The listing builds one solid part. Answer for the finished solid, in the listing's coordinates (mm). Coordinates: 2 decimals unless noted, no trailing zeros. Order: outer loops, then holes, each group sorted by start corner. A loop starts at its lowest first (then second) coordinate and runs counter-clockwise, first axis right, second up.
Autodesk Inventor part; units mm, degrees
ref_plane "YZ Plane" through (0, 0, 0) normal (1, 0, 0) x (0, 1, 0)
ref_plane "XZ Plane" through (0, 0, 0) normal (0, 1, 0) x (-1, 0, 0)
ref_plane "XY Plane" through (0, 0, 0) normal (0, 0, 1) x (1, 0, 0)
sketch "Sketch1" plane through (0, 0, 0) normal (0, 1, 0) x (-1, 0, 0)
  line L0 (0, 0) -> (-140, 0)
  line L1 (-140, 0) -> (-140, -120)
  line L2 (-140, -120) -> (0, -120)
  line L3 (0, -120) -> (0, 0)
  line L4 (-25, 0) -> (-75, 0)
  line L5 (-75, 0) -> (-75, -20)
  line L6 (-75, -20) -> (-25, -20)
  line L7 (-25, -20) -> (-25, 0)
  circle A0 centre (-5, -5) radius 1.6
  circle A1 centre (-10, -5) radius 1.6
  circle A2 centre (-15, -5) radius 1.6
  circle A3 centre (-20, -5) radius 1.6
  circle A4 centre (-130, -30) radius 1.6
  line L8 (0, -60) -> (-140, -60) construction
  line L9 (-70, -120) -> (-70, 0) construction
  circle A5 centre (-135, -5) radius 1.6
  circle A6 centre (-130, -5) radius 1.6
  circle A7 centre (-125, -5) radius 1.6
  circle A8 centre (-120, -5) radius 1.6
  circle A9 centre (-130, -60) radius 1.6
  circle A10 centre (-130, -30) radius 2.75
  circle A11 centre (-130, -60) radius 2.75
  circle A12 centre (-5, -115) radius 1.6
  circle A13 centre (-10, -115) radius 1.6
  circle A14 centre (-30, -110) radius 1.6
  circle A15 centre (-30, -110) radius 2.75
  circle A16 centre (-110, -110) radius 1.6
  circle A17 centre (-110, -110) radius 2.75
  circle A18 centre (-70, -110) radius 1.6
  circle A19 centre (-70, -110) radius 2.75
  circle A20 centre (-44, -38) radius 1.6
  circle A21 centre (-44, -38) radius 2.75
  circle A22 centre (-56, -38) radius 1.6
  circle A23 centre (-56, -38) radius 2.75
  circle A24 centre (-57.5, -60) radius 1.6
  circle A25 centre (-57.5, -60) radius 2.75
  circle A26 centre (-57.5, -72) radius 1.6
  circle A27 centre (-57.5, -72) radius 2.75
  circle A28 centre (-42.5, -60) radius 1.6
  circle A29 centre (-42.5, -60) radius 2.75
  circle A30 centre (-42.5, -72) radius 1.6
  circle A31 centre (-42.5, -72) radius 2.75
  circle A32 centre (-10, -30) radius 1.6
  circle A33 centre (-10, -60) radius 1.6
  circle A34 centre (-10, -30) radius 2.75
  circle A35 centre (-10, -60) radius 2.75
  circle A36 centre (-10, -90) radius 1.6
  circle A37 centre (-10, -90) radius 2.75
  circle A38 centre (-80, -2.5) radius 1.6
  circle A39 centre (-80, -17.5) radius 1.6
  circle A40 centre (-105, -10) radius 1.6
  circle A41 centre (-105, -20) radius 1.6
  circle A42 centre (-95, -20) radius 1.6
  circle A43 centre (-95, -10) radius 1.6
  circle A44 centre (-95, -30) radius 1.6
  circle A45 centre (-95, -40) radius 1.6
  circle A46 centre (-105, -30) radius 1.6
  circle A47 centre (-105, -40) radius 1.6
  circle A48 centre (-95, -50) radius 1.6
  circle A49 centre (-95, -60) radius 1.6
  circle A50 centre (-105, -50) radius 1.6
  circle A51 centre (-105, -60) radius 1.6
  circle A52 centre (-110, -80) radius 1.65
  circle A53 centre (-110, -80) radius 2.75
  circle A54 centre (-70, -80) radius 1.65
  circle A55 centre (-70, -80) radius 2.75
  circle A56 centre (-30, -80) radius 1.65
  circle A57 centre (-30, -80) radius 2.75
  line L10 (0, -120) -> (-15, -120)
  line L11 (-15, -120) -> (-15, -100)
  line L12 (-15, -100) -> (0, -100)
  line L13 (0, -100) -> (0, -120)
  circle A58 centre (-90, -110) radius 1.6
  point P0 (-50, -38)
  point P1 (-50, -74.6125)
  dimension "d0" = 140
  dimension "d1" = 120
  dimension "d2" = 50
  dimension "d3" = 20
  dimension "d4" = 25
  dimension "d5" = 3.2
  dimension "d6" = 5
  dimension "d7" = 5
  dimension "d8" = 3.2
  dimension "d9" = 5
  dimension "d10" = 3.2
  dimension "d11" = 5
  dimension "d12" = 3.2
  dimension "d13" = 5
  dimension "d14" = 3.2
  dimension "d15" = 10
  dimension "d16" = 30
  dimension "d17" = 3.2
  dimension "d18" = 5.5
  dimension "d19" = 5.5
  dimension "d20" = 3.2
  dimension "d22" = 5.5
  dimension "d23" = 3.2
  dimension "d24" = 5.5
  dimension "d28" = 3.2
  dimension "d30" = 5.5
  dimension "d34" = 3.2
  dimension "d37" = 5.5
  dimension "d42" = 30
  dimension "d43" = 10
  dimension "d44" = 10
  dimension "d46" = 10
  dimension "d47" = 3.2
  dimension "d48" = 5
  dimension "d49" = 2.5
  dimension "d50" = 3.2
  dimension "d51" = 15
  dimension "d52" = 3.2
  dimension "d53" = 3.2
  dimension "d54" = 10
  dimension "d55" = 3.2
  dimension "d56" = 10
  dimension "d57" = 3.2
  dimension "d58" = 20
  dimension "d59" = 10
  dimension "d60" = 10
  dimension "d61" = 3.2
  dimension "d62" = 10
  dimension "d63" = 3.2
  dimension "d64" = 10
  dimension "d65" = 3.2
  dimension "d66" = 3.2
  dimension "d67" = 3.2
  dimension "d68" = 10
  dimension "d69" = 3.2
  dimension "d70" = 10
  dimension "d71" = 3.2
  dimension "d72" = 3.2
  dimension "d73" = 3.3
  dimension "d74" = 5.5
  dimension "d76" = 3.3
  dimension "d77" = 5.5
  dimension "d78" = 30
  dimension "d79" = 30
extrude "Extrusion1" add sketch "Sketch1" along normal blind 4 contours L3 L12 L11 L2 L1 L0 L5 L6 L7
extrude "Extrusion2" add sketch "Sketch1" along normal blind 2 contours A10 | A11 | A15 | A17 | A19 | A21 | A23 | A25 | A27 | A29 | A31 | A34 | A35 | A37 | A53 | A55 | A57
fillet "Fillet1" radius 5 7 edges at (15, 2, -100) (0, 2, -100) (75, 2, 0) (25, 2, 0) (0, 2, 0) (75, 2, -20) (25, 2, -20)
properties part number "Fix Casis Kiri Depan_3DPrint"
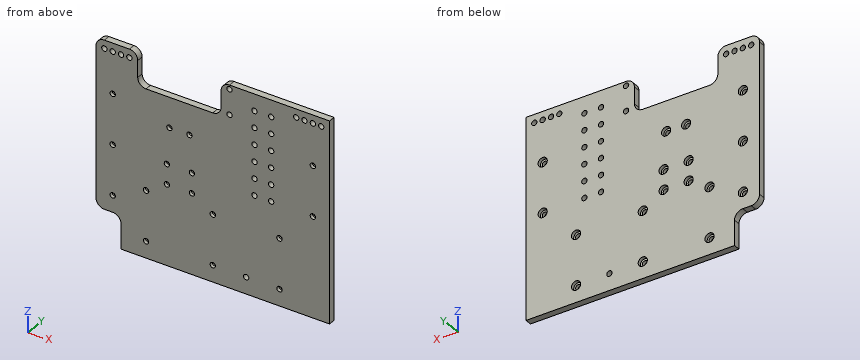
(1) Find section C-C on x = 135. Determine the outline of the cut face in (y, z).
(2) Find section D-D on z = -30. Determine the outline of the cut face in (x, y).
(3) Given pin 1 Ø3 at (x, z) = (41.5, -60) entering from +Y, flat-ended and moving along its own axis, determine where the tip first touches the part or whether it passes through.
(4) Find section B-B on z = -90. Determine the outline of the cut face in (x, y), then the cut area to 3 significant figures.
(5) Find the intervals of material crossed by probe 1 along Z at (x, y) = (70, 1.45); probe 2 along X at (y, z) = (1.5, -72.5); probe 3 along X at (y, z) = (2.8, -81), in increasing order.
(6) Find section A-A on x = 110. Determine the outline of the cut face in (y, z), then the cut area to 3 significant figures.
Resolved:
1. outline: (0, -120) - (4, -120) - (4, -6.6) - (0, -6.6) - close; (0, -3.4) - (4, -3.4) - (4, 0) - (0, 0) - close
2. outline: (0, 0) - (8.4, 0) - (8.4, 2) - (7.25, 2) - (7.25, 4) - (0, 4) - close; (11.6, 0) - (93.4, 0) - (93.4, 4) - (12.75, 4) - (12.75, 2) - (11.6, 2) - close; (96.6, 0) - (103.4, 0) - (103.4, 4) - (96.6, 4) - close; (106.6, 0) - (128.4, 0) - (128.4, 2) - (127.25, 2) - (127.25, 4) - (106.6, 4) - close; (131.6, 0) - (140, 0) - (140, 4) - (132.75, 4) - (132.75, 2) - (131.6, 2) - close
3. pin 1: stops at y = 2
4. outline: (0, 0) - (8.4, 0) - (8.4, 2) - (7.25, 2) - (7.25, 4) - (0, 4) - close; (11.6, 0) - (140, 0) - (140, 4) - (12.75, 4) - (12.75, 2) - (11.6, 2) - close
4. area: 543 mm2
5. probe 1: z = -120 to -111.6, -108.4 to -81.65, -78.35 to -20
5. probe 2: x = 0 to 40.98, 44.02 to 55.98, 59.02 to 140
5. probe 3: x = 0 to 27.44, 32.56 to 67.44, 72.56 to 107.44, 112.56 to 140
6. outline: (0, -120) - (4, -120) - (4, -112.75) - (2, -112.75) - (2, -111.6) - (0, -111.6) - close; (0, -108.4) - (2, -108.4) - (2, -107.25) - (4, -107.25) - (4, -82.75) - (2, -82.75) - (2, -81.65) - (0, -81.65) - close; (0, -78.35) - (2, -78.35) - (2, -77.25) - (4, -77.25) - (4, 0) - (0, 0) - close
6. area: 445 mm2
